CAD build for the part. Positions are in the model's coordinates, mm. Give positions to 0.01 mm unless a question says otherwise; leave off trailing zeros. Write each loop counter-clockwise with the first axis right and the second up, starting at its lowest first coordinate (ties: lowest second). Pieces come first, ordered by that corner, then holes. Notation, with made-up numbers: (66, 45.5) -> (118, 45.5) arc R19 ccw to (118, 67.5) -> close; hole circle Ø3 at (-5, 23). An arc over 180 degrees is marked (long way). Answer as a JSON object with one key per item and string values.
Autodesk Inventor part; units mm, degrees
ref_plane "YZ Plane" through (0, 0, 0) normal (1, 0, 0) x (0, 1, 0)
ref_plane "XZ Plane" through (0, 0, 0) normal (0, 1, 0) x (-1, 0, 0)
ref_plane "XY Plane" through (0, 0, 0) normal (0, 0, 1) x (1, 0, 0)
sketch "Boceto1" plane through (0, 0, 0) normal (0, 0, 1) x (1, 0, 0)
  line L0 (-65, -50) -> (65, -50)
  line L1 (65, -50) -> (65, 50)
  line L2 (65, 50) -> (-65, 50)
  line L3 (-65, 50) -> (-65, -50)
  line L4 (-65, -50) -> (65, 50) construction
  line L5 (65, -50) -> (-65, 50) construction
  line L6 (-50, -35) -> (50, -35)
  line L7 (50, -35) -> (50, 35)
  line L8 (50, 35) -> (-50, 35)
  line L9 (-50, 35) -> (-50, -35)
  line L10 (-50, -35) -> (50, 35) construction
  line L11 (50, -35) -> (-50, 35) construction
  point P0 (0, 0)
  dimension "d0" = 130
  dimension "d1" = 100
  dimension "d2" = 100
  dimension "d3" = 70
extrude "Extrusión1" add sketch "Boceto1" along normal blind 5.5
sketch "Boceto2" plane through (0, 0, 0) normal (0, 0, 1) x (1, 0, 0)
  line L0 (0, 0) -> (-20, 0)
  line L1 (-20, 0) -> (-20, 35)
  line L2 (-50, 35) -> (50, 35)
  line L3 (-20, 0) -> (0, 0)
  line L4 (0, 0) -> (0, 35)
  line L5 (0, 35) -> (-20, 35)
  line L6 (-20, 35) -> (-20, 0)
  line L7 (50, -35) -> (-50, -35)
  line L8 (-20, 0) -> (0, 0)
  line L9 (0, 0) -> (0, -35)
  line L10 (0, -35) -> (-20, -35)
  line L11 (-20, -35) -> (-20, 0)
  line L12 (50, 35) -> (40, 35)
  line L13 (40, 35) -> (40, -35)
  line L14 (50, 35) -> (50, -35)
  line L15 (50, -35) -> (50, 35)
  line L16 (50, -35) -> (40, -35)
  dimension "d6" = 20
  dimension "d7" = 10
extrude "Extrusión9" add sketch "Boceto2" along normal blind 5.5 contours L9 L7 L11 L0 | L0 L1 L2 L4 | L2 L14 L7 L13
sketch "Boceto8" plane through (0, 0, 5.5) normal (0, 0, 1) x (1, 0, 0)
  line L0 (0, 0) -> (-20, 0)
  line L1 (-20, 35) -> (-20, -35)
  line L2 (-10, 0) -> (-10, 50)
  line L3 (65, 50) -> (-65, 50)
  line L4 (0, 35) -> (-10, 35)
  line L5 (-10, 35) -> (-10, 50)
  line L6 (-10, 50) -> (-10, 42.5)
  line L7 (-10, 0) -> (65, 0)
  line L8 (65, -50) -> (65, 50)
  line L9 (40, 35) -> (40, -35)
  line L10 (40, 0) -> (65, 0)
  line L11 (52.5, 0) -> (52.5, 20)
  circle A0 centre (-10, 42.5) radius 3
  circle A1 centre (52.5, 20) radius 3
  circle A2 centre (-10, -42.5) radius 3
  circle A3 centre (52.5, -20) radius 3
  dimension "d32" = 20
  dimension "d33" = 6
  dimension "d34" = 6
extrude "Extrusión10" cut sketch "Boceto8" against normal blind 5.5 contours A1 | A0 L2 | L2 A0 | A2 | A3
sketch "Boceto9" plane through (0, 0, 5.5) normal (0, 0, 1) x (1, 0, 0)
  line L0 (-20, 35) -> (-20, -35)
  line L1 (-20, 0) -> (0, 0)
  circle A0 centre (-10, 0) radius 25
  dimension "d40" = 50
extrude "Extrusión12" add sketch "Boceto9" against normal blind 5.5
properties part number "BASE"
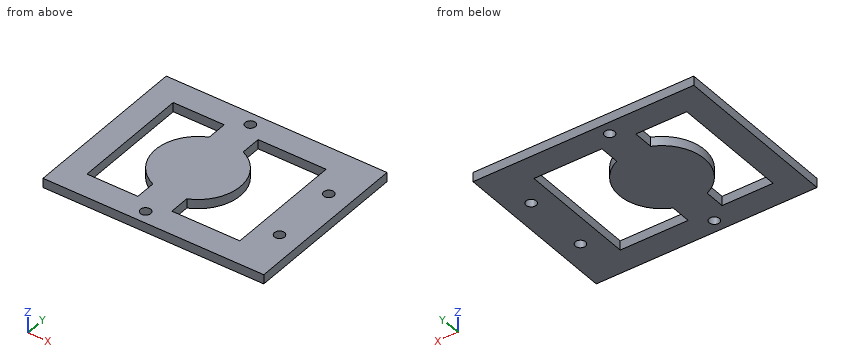
1) Pin check, flat tip, straight feed: pin 1 (3.5 mm diameter, centred on x = -10, y = -42.5, fed in from -Z). Stop position of the tip, or through.
Model answer:
{"pin 1": "passes through"}
2) Slice it at B-B (y = 20). List the corners of the cut face in (x, z).
Model answer:
{"outline": "(-65, 0) -> (-50, 0) -> (-50, 5.5) -> (-65, 5.5) -> close; (-25, 0) -> (5, 0) -> (5, 5.5) -> (-25, 5.5) -> close; (40, 0) -> (49.5, 0) -> (49.5, 5.5) -> (40, 5.5) -> close; (55.5, 0) -> (65, 0) -> (65, 5.5) -> (55.5, 5.5) -> close"}
3) Wall check: probe 1 along Y at (x, z) = (52.5, 4); probe 2 along Y at (x, z) = (-10, 2.1); probe 3 along X at (y, z) = (42.5, 2.65). Give the ranges that are in metal, low to high.
Model answer:
{"probe 1": "y = -50 to -23, -17 to 17, 23 to 50", "probe 2": "y = -50 to -45.5, -39.5 to 39.5, 45.5 to 50", "probe 3": "x = -65 to -13, -7 to 65"}
4) Slice it at A-A (y = -42.5). List the corners of the cut face in (x, z).
Model answer:
{"outline": "(-65, 0) -> (-13, 0) -> (-13, 5.5) -> (-65, 5.5) -> close; (-7, 0) -> (65, 0) -> (65, 5.5) -> (-7, 5.5) -> close"}
5) Slice it at C-C (z = 0.9). List the corners of the cut face in (x, y), then the cut area to 3 significant figures.
Model answer:
{"outline": "(-65, -50) -> (65, -50) -> (65, 50) -> (-65, 50) -> close; hole (-50, -35) -> (-20, -35) -> (-20, -22.91) arc R25 cw to (-20, 22.91) -> (-20, 35) -> (-50, 35) -> close; hole circle Ø6 at (-10, -42.5); hole circle Ø6 at (-10, 42.5); hole (0, -35) -> (40, -35) -> (40, 35) -> (0, 35) -> (0, 22.91) arc R25 cw to (0, -22.91) -> close; hole circle Ø6 at (52.5, -20); hole circle Ø6 at (52.5, 20)", "area": "8,980 mm2"}
6) Slice it at D-D (x = -10). List the corners of the cut face in (y, z), then the cut area to 3 significant figures.
Model answer:
{"outline": "(-50, 0) -> (-45.5, 0) -> (-45.5, 5.5) -> (-50, 5.5) -> close; (-39.5, 0) -> (39.5, 0) -> (39.5, 5.5) -> (-39.5, 5.5) -> close; (45.5, 0) -> (50, 0) -> (50, 5.5) -> (45.5, 5.5) -> close", "area": "484 mm2"}
